Autodesk Inventor part; units mm, degrees
ref_plane "YZ Plane" through (0, 0, 0) normal (1, 0, 0) x (0, 1, 0)
ref_plane "XZ Plane" through (0, 0, 0) normal (0, 1, 0) x (-1, 0, 0)
ref_plane "XY Plane" through (0, 0, 0) normal (0, 0, 1) x (1, 0, 0)
sketch "Sketch1" plane through (0, 0, 0) normal (0, 0, 1) x (1, 0, 0)
  circle A0 centre (0, 0) radius 2.55
  circle A1 centre (0, 0) radius 5.5
  dimension "d0" = 5.1
  dimension "d1" = 11
extrude "Extrusion1" add sketch "Sketch1" along normal blind 8
chamfer "Chamfer1" distance 1.75 distance2 2.5 1 edges at (-5.5, 0, 8) measured on face at (4.4387, -0.6422, 8)
sketch "Sketch2" plane through (0, 0, 0) normal (0, 1, 0) x (-1, 0, 0)
  line L0 (-5.5, 0) -> (5.5, 0)
  line L1 (5.5, 5.5) -> (-5.5, 5.5)
  line L2 (-5.5, 0) -> (-5.5, 5.5)
  line L3 (5.5, 0) -> (5.5, 5.5)
  point P0 (0, 0)
  point P1 (0, 2.75)
  dimension "d7" = 11
  dimension "d8" = 5.5
  dimension "d9" = 5.5
  dimension "d10" = 2.75
hole "Hole1" at (0, 0, 2.75) direction (0, 1, 0) diameter 2.5 end through all both
properties part number "3DP_PLA_X_axis_idler_shaft_locking_ring"
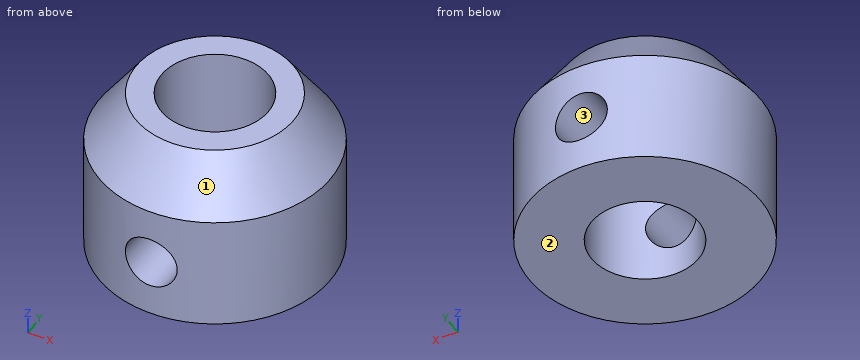
CAD build for the part. Positions are in the model's coordinates, mm. Face numbers are marked on the shaded views. Coordinates: 2 decimals unless noted, no trailing zeros. Order: outer loops, then holes, each group sorted by start corner. A loop starts at its lowest first (then second) coordinate and runs counter-clockwise, first axis right, second up.
Item 1: Band-saw the part on C-C on z = 2.75. List the corners of the cut face in (x, y).
Check sheet entries:
outline: (-1.25, -5.36) - (-1.25, -2.22) arc R2.55 cw to (-1.25, 2.22) - (-1.25, 5.36) arc R5.5 ccw to start; (1.25, -5.36) arc R5.5 ccw to (1.25, 5.36) - (1.25, 2.22) arc R2.55 cw to (1.25, -2.22) - close
Item 2: Drill centre lines: L1, parallel to Z at x = 0, y = -3.55; L2, parallel to X at y = -4, z = 2.75; L3, parallel to Y at x = 2, z = 2. Where is each one in solid material? Low to high.
Check sheet entries:
L1: z = 0 to 1.5, 4 to 8
L2: x = -3.77 to -1.25, 1.25 to 3.77
L3: y = -5.12 to -1.58, 1.58 to 5.12
Item 3: Two-plate mould, pull along Z, no slides. Class the marked faces 1, 2 and 3: +Z half, -Z half, draft (parallel to the pull), parting line (faces both ways), or undercut.
Check sheet entries:
face 1: +Z half
face 2: -Z half
face 3: undercut
Item 4: Band-saw the part on A-A on x = 0. List the corners of the cut face in (y, z).
Check sheet entries:
outline: (-5.5, 0) - (-2.55, 0) - (-2.55, 1.5) - (-5.5, 1.5) - close; (-5.5, 4) - (-2.55, 4) - (-2.55, 8) - (-3.75, 8) - (-5.5, 5.5) - close; (2.55, 0) - (5.5, 0) - (5.5, 1.5) - (2.55, 1.5) - close; (2.55, 4) - (5.5, 4) - (5.5, 5.5) - (3.75, 8) - (2.55, 8) - close
Item 5: Band-saw the part on B-B on y = 0. List the corners of the cut face in (x, z).
Check sheet entries:
outline: (-5.5, 0) - (-2.55, 0) - (-2.55, 8) - (-3.75, 8) - (-5.5, 5.5) - close; (2.55, 0) - (5.5, 0) - (5.5, 5.5) - (3.75, 8) - (2.55, 8) - close
Item 6: Band-saw the part on D-D on z = 1. List the corners of the cut face in (x, y), plus the area to 3 significant figures.
Check sheet entries:
outline: circle Ø11 at (0, 0); hole circle Ø5.1 at (0, 0)
area: 74.6 mm2
Item 7: Pin check, flat tip, straight feed: pin 1 Ø3 at (x, z) = (3, 6) entering from -Y. Stop position of the tip, or through.
Check sheet entries:
pin 1: stops at y = -5.27
